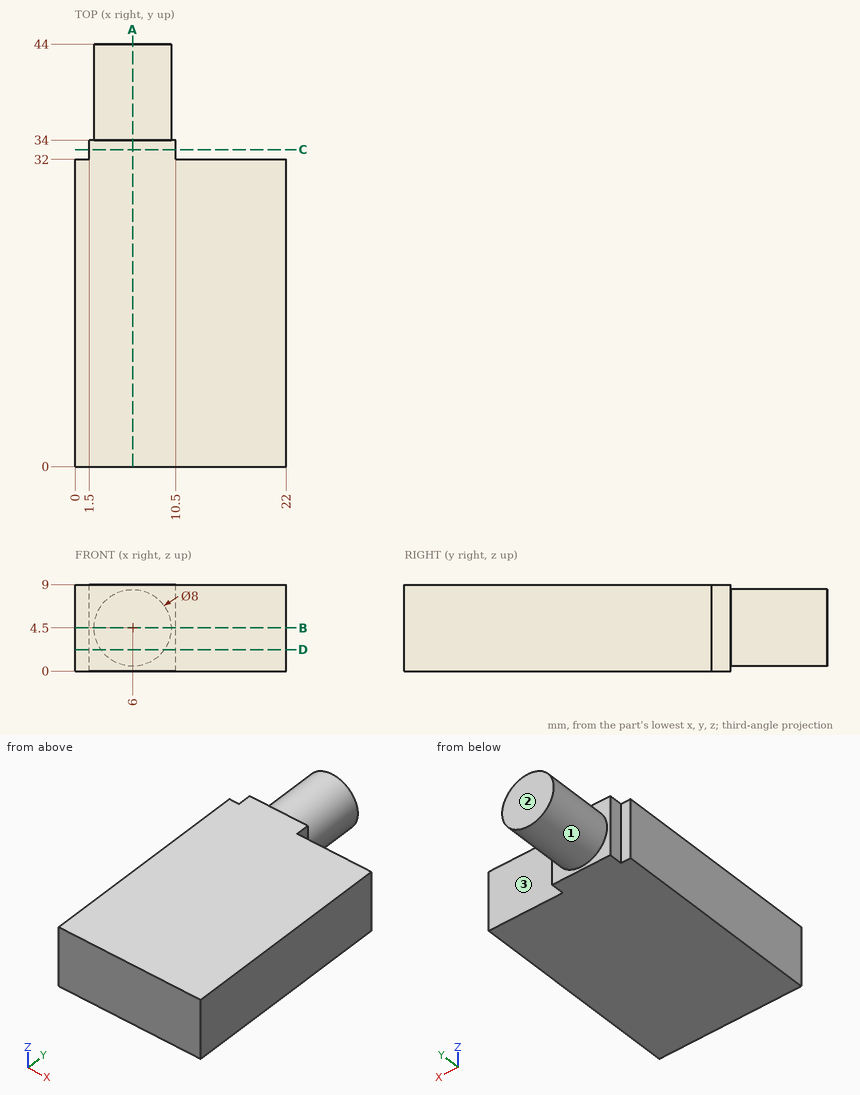
For this review, use the dimensioned drawing (mm, ordinates from the lowest corner) and the shaded views. A direction names the side the tool comes from. Coordinates: 2 decimals unless noted, no trailing zeros. Write each loop counter-clockwise with the first axis right and the second up, starting at its lowest first coordinate (ties: lowest second). Pieces come first, ordered by that corner, then holes. Notation, with made-up numbers: (-7, -2) -> (49, -2) arc R8 ccw to (49, 4) -> close; hole circle Ø6 at (33.25, -35). An arc over 180 degrees is marked (long way). Put each result on its own line as item: value.
Q1. Tool access review of the marked faces 1, 2 and 3: name each direction out of +Z, -Z, +X, -X, +Y, -Y from which nothing blocks a thin tool from reaching the whole face with its end or side.
From the geometry:
face 1: +Y
face 2: +Z, -Z, +X, -X, +Y
face 3: +Z, -Z, +X, +Y
Q2. Clearance check with flat-ended pins moving along their axes: pin 1 Ø1 at (y, z) = (33, 3.5) entering from +X; pin 2 Ø0.6 at (y, z) = (33.5, 6.5) entering from -X; pin 3 Ø1.2 at (x, z) = (1, 4.5) entering from +Y. State where each tip first meets the part, or that it passes through.
From the geometry:
pin 1: stops at x = 10.5
pin 2: stops at x = 1.5
pin 3: stops at y = 34
Q3. Take a section at D-D, the plane z = 2.25. State the section outline as (x, y) points.
From the geometry:
outline: (0, 0) -> (22, 0) -> (22, 32) -> (10.5, 32) -> (10.5, 34) -> (9.31, 34) -> (9.31, 44) -> (2.69, 44) -> (2.69, 34) -> (1.5, 34) -> (1.5, 32) -> (0, 32) -> close
Q4. Wall thickness on L1, parallel to Y at x = 17.75, z = 5.5; L2, parallel to Y at x = 3.5, z = 1.25; L3, parallel to X at y = 34.5, z = 7: over which ranges is each line inside the solid? List them lowest first.
From the geometry:
L1: y = 0 to 32
L2: y = 0 to 34
L3: x = 2.88 to 9.12
Q5. Take a section at A-A, the plane x = 6. State the section outline as (y, z) points, then the cut area to 3 significant figures.
From the geometry:
outline: (0, 0) -> (34, 0) -> (34, 0.5) -> (44, 0.5) -> (44, 8.5) -> (34, 8.5) -> (34, 9) -> (0, 9) -> close
area: 386 mm2
Q6. Take a section at C-C, the plane y = 33. State the section outline as (x, z) points, then the cut area to 3 significant figures.
From the geometry:
outline: (1.5, 0) -> (10.5, 0) -> (10.5, 9) -> (1.5, 9) -> close
area: 81.0 mm2
Q7. Take a section at B-B, the plane z = 4.5. State the section outline as (x, y) points, then the cut area to 3 significant figures.
From the geometry:
outline: (0, 0) -> (22, 0) -> (22, 32) -> (10.5, 32) -> (10.5, 34) -> (10, 34) -> (10, 44) -> (2, 44) -> (2, 34) -> (1.5, 34) -> (1.5, 32) -> (0, 32) -> close
area: 802 mm2
